Could you check a few things on this model? Use its own coordinates, in mm. A direction names the side the tool comes from. Round coordinates to 2 decimals unless told otherwise and drop trailing zeros. Write each loop counter-clockwise with the first axis right and the second up, starting at its lowest first coordinate (ties: lowest second). Pieces come first, ordered by that corner, then holes. Notation, with made-up numbers: (-22.75, 78) -> (10.25, 78) arc R22 cw to (10.25, 99) -> close; hole circle Ø6 at (70.5, 77). An arc over 180 degrees is marked (long way). Return JSON: item names as keys, results as strings.
from build123d import *

# Parameters (mm, degrees)
BOSS_EXTRUDE1_DEPTH = 30
SKETCH2_R           = 30
BOSS_EXTRUDE2_DEPTH = 29
SKETCH1_3_R         = 10
CUT_EXTRUDE1_DEPTH  = 30
BOSS_EXTRUDE3_START = -59
SKETCH1_4_R         = 18
BOSS_EXTRUDE3_DEPTH = 47
SKETCH3_W           = 60
SKETCH3_H           = 15
CUT_EXTRUDE2_DEPTH  = 45


with BuildPart() as part:
    # Sketch1 → Boss-Extrude1 (new body)
    with BuildSketch(Plane.XY):
        with BuildLine():
            Line((-182.5, 30), (182.5, 30))
            ThreePointArc((182.5, 30), (212.5, 0), (182.5, -30))
            Line((182.5, -30), (-182.5, -30))
            ThreePointArc((-182.5, -30), (-212.5, 0), (-182.5, 30))
        make_face()
    extrude(amount=-BOSS_EXTRUDE1_DEPTH)

    # Sketch2 → Boss-Extrude2 (add)
    with BuildSketch(Plane(origin=(0, 0, -30), x_dir=(-1, 0, 0), z_dir=(0, 0, -1))):
        with Locations((-182.5, 0)):
            Circle(SKETCH2_R)
        with Locations((182.5, 0)):
            Circle(SKETCH2_R)
    extrude(amount=BOSS_EXTRUDE2_DEPTH)

    # Sketch1<3> → Cut-Extrude1 (cut)
    with BuildSketch(Plane.XY):
        Circle(SKETCH1_3_R)
    extrude(amount=-CUT_EXTRUDE1_DEPTH, mode=Mode.SUBTRACT)

    # Sketch1<4> → Boss-Extrude3 (add)
    with BuildSketch(Plane.XY.offset(BOSS_EXTRUDE3_START)):
        with Locations((182.5, 0)):
            Circle(SKETCH1_4_R)
        with Locations((-182.5, 0)):
            Circle(SKETCH1_4_R)
    extrude(amount=-BOSS_EXTRUDE3_DEPTH)

    # Sketch3 → Cut-Extrude2 (cut)
    with BuildSketch(Plane.XZ.offset(30)):
        with Locations((0, -15)):
            Rectangle(SKETCH3_W, SKETCH3_H)
    extrude(amount=-CUT_EXTRUDE2_DEPTH, mode=Mode.SUBTRACT)


solid = part.part
1) I want a section at A-A, the plane x = -17.5. Please give me the cut outline in (y, z).
Return value:
{"outline": "(-30, -30) -> (30, -30) -> (30, 0) -> (-30, 0) -> (-30, -7.5) -> (15, -7.5) -> (15, -22.5) -> (-30, -22.5) -> close"}
2) Thinking about a two-plate mould opening in Z: for faces 1 (the face through (3, 14, 0)), 2 (the face through (0, -13, -22.5)), 3 (the face through (-2.17, -9.76, -26.2)), 4 (the face through (0, -13, -7.5)), which applies, pulls with the +Z half, pulls with the -Z half, needs draft (parallel to the pull), parting line crosses it, or undercut?
Return value:
{"face 1": "pulls with the +Z half", "face 2": "undercut", "face 3": "needs draft", "face 4": "undercut"}
3) I want a section at B-B, the plane z = -14. Please give me the cut outline in (x, y).
Return value:
{"outline": "(-182.5, -30) -> (-30, -30) -> (-30, 15) -> (30, 15) -> (30, -30) -> (182.5, -30) arc R30 ccw to (182.5, 30) -> (-182.5, 30) arc R30 ccw to start"}
4) I want a section at C-C, the plane z = -88.5. Please give me the cut outline in (x, y), and give its area (3 significant figures).
Return value:
{"outline": "circle Ø36 at (-182.5, 0); circle Ø36 at (182.5, 0)", "area": "2,040 mm²"}
5) If I drill on probe 1 along Y at (x, z) = (0, -4.5); probe 2 along Z at (x, y) = (10, -25); probe 3 along Z at (x, y) = (-107, 19), over which ranges is the centre line in solid material (lowest first)? Write a range as [from, to].
Return value:
{"probe 1": "[-30, -10], [10, 30]", "probe 2": "[-30, -22.5], [-7.5, 0]", "probe 3": "[-30, 0]"}
6) For faces 5 (the face through (-30, -8, -15)), 6 (the face through (-195.4, -12.9, -59)), 7 (the face through (-2.17, -9.76, -3.7)), which set-ups out of +Z, -Z, +X, -X, +Y, -Y let a thin tool reach every point of the face, with its end or its side?
Return value:
{"face 5": "-Y", "face 6": "-Z", "face 7": "+Z, -Z"}
7) Will these pins go through, and if not, where does the flat tip stop? pin 1 Ø1 at (y, z) = (-23.5, -16.5) entering from -X; pin 2 Ø16.5 at (y, z) = (-11.5, -11.5) entering from -X; pin 3 Ø8 at (y, z) = (16.5, -56.5) entering from -X; pin 4 Ø18 at (x, y) = (0, 0) entering from -Z (1 decimal).
Return value:
{"pin 1": "x = -201.76", "pin 2": "x = -212.32", "pin 3": "x = -209.77", "pin 4": "through"}
8) I want a section at D-D, the plane x = 73. Please give me the cut outline in (y, z).
Return value:
{"outline": "(-30, -30) -> (30, -30) -> (30, 0) -> (-30, 0) -> close"}
